Answer from the drawing. Dimensions are ordinates in mm from the lowest x, y and z of the part. Coordinates: 2 decimals unless noted, no trailing zeros. Loops run counter-clockwise (first coordinate to the right, second up) from the corner with the lowest first, then second, coordinate; pieces in that order, holes last. Notation, with made-up numbers: (-17, 20) - (14, 20) arc R14 ccw to (14, 34) - close; hole circle Ø1 at (-24.5, 70.5). An arc over 180 degrees is marked (long way). Write each question's results on one line, items separated by ' | '. Start each with the question number.
1. A cutting plane is placed at C-C on x = 40.5. Determine the outline of the cut face in (y, z).
2. This flat-tipped pin is pushed along its axis until it touches: P1, Ø1, axis at x = 37, z = 6, coming from the +Y side. Where does it stop, or does it pass through?
3. Find the intervals of material crossed by line 1 along X through (y, z) = (0.8, 19) (3 decimals); line 2 along Y through (x, z) = (67, 20); line 3 along Z through (x, y) = (101.5, 9), in increasing order. Write a range as [from, to].
4. A cutting plane is placed at B-B on y = 9. Determine the outline of the cut face in (x, z), then the cut area to 3 significant figures.
5. Determine the mould class of the marked faces 1 and 2 for opening direction Y: released by +Y, released by -Y, zero draft, split by the parting line, or undercut.
6. A cutting plane is placed at A-A on z = 3.5. Determine the outline of the cut face in (x, y).
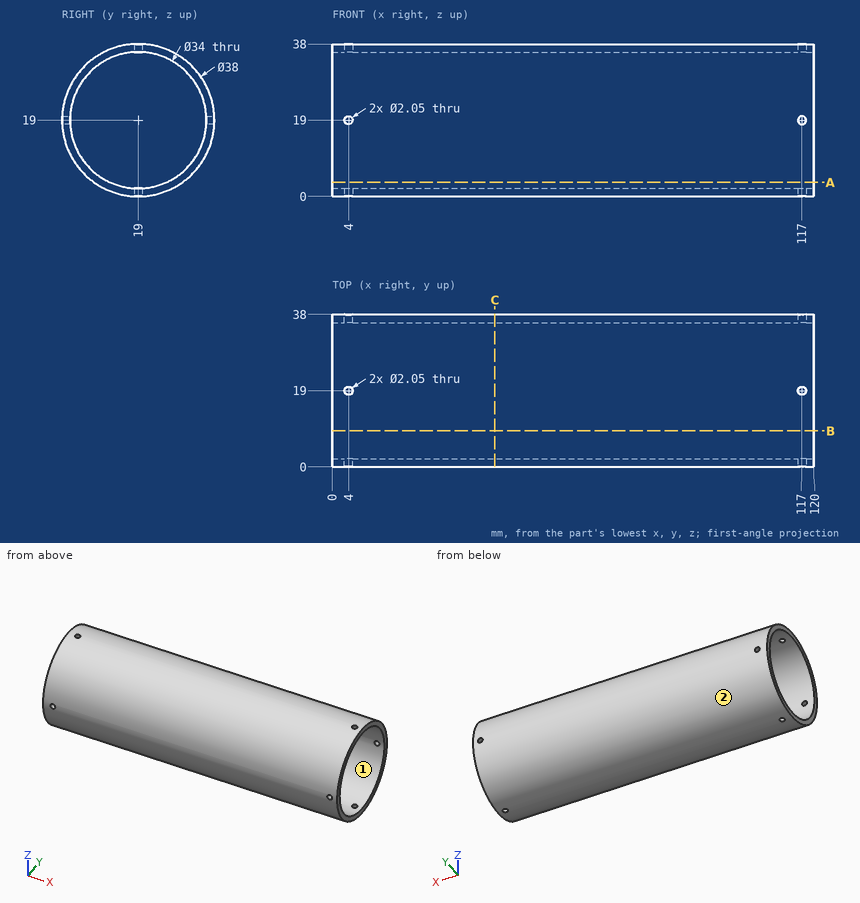
Values:
1) outline: circle Ø38 at (19, 19); hole circle Ø34 at (19, 19)
2) P1: y = 33.31
3) line 1: [0, 2.975], [5.025, 115.975], [118.025, 120] | line 2: [0.03, 2.03], [35.97, 37.97] | line 3: [2.84, 5.25], [32.75, 35.16]
4) outline: (0, 2.84) - (120, 2.84) - (120, 5.25) - (0, 5.25) - close; (0, 32.75) - (120, 32.75) - (120, 35.16) - (0, 35.16) - close | area: 578 mm^2
5) face 1: undercut | face 2: split by the parting line
6) outline: (0, 8.01) - (120, 8.01) - (120, 12.02) - (0, 12.02) - close; (0, 25.98) - (120, 25.98) - (120, 29.99) - (0, 29.99) - close
